Part model, mm, in its own coordinate system. Face numbers are marked on the shaded views. A direction names the side the tool comes from. Round coordinates to 2 decimals unless told otherwise and drop trailing zeros. Loops run counter-clockwise (first coordinate to the right, second up) from the corner with the lowest first, then second, coordinate; pieces in that order, holes last. Notation, with made-up numbers: M 73,73.25 L 100,73.25 A22 cw 100,98.25 Z; hole C 76,-30 d5. An arc over 180 degrees is marked long. Put each result on its own line as item: value. Start each with the question number.
1) Which spindle directions (+Z, -Z, +X, -X, +Y, -Y) get a long thin tool onto all of the face, cutting with end or side? Do the marked faces 5 and 6. Say none if no direction does.
2) Drop flat-ended pins along their axis: pin 1 Ø4 at (x, z) = (42, 7.5) entering from +Y; pin 2 Ø5 at (x, z) = (3, 2) entering from +Y; pin 3 Ø6 at (y, z) = (-1.5, 5.5) entering from +X; pin 4 Ø6.5 at (x, y) = (-64, 10) entering from +Z. Give the stop position or say it passes through.
3) Pull direction Y, two halves, no side cores. Call the marked faces 1, 2, 3 and 4: +Y half, -Y half, draft (parallel to the pull), parting line (faces both ways), or undercut.
4) Slice it at A-A on x = -9.5. Give the cut face in (y, z), then the cut area to 3 significant figures.
5) Probe line 1 along X through (y, z) = (10, 6); line 2 along X through (y, z) = (10, 9.75); line 3 along X through (y, z) = (7.25, 2.25). List the from-to ranges inside material, lowest first.
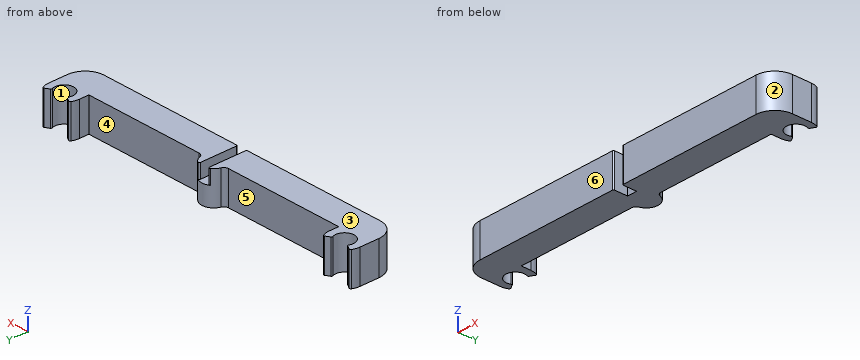
```python
from build123d import *

# Parameters (mm, degrees)
F1_DEPTH = 14
F2_W     = 4.1
F2_H     = 18.371435
F3_DEPTH = 6
F4_R     = 8
F5_R     = 0.5
F6_R     = 2


with BuildPart() as f1:
    # F0 (on Top) → F1 (new body)
    with BuildSketch(Plane.XY):
        with BuildLine():
            Line((-71, -6), (-2.05, -6))
            Line((-2.05, -6), (-2.05, 0))
            Line((-2.05, 0), (-2.05, 6))
            Line((-2.05, 6), (-5, 6))
            Line((-5, 6), (-57, 6))
            Line((-57, 6), (-57, 10))
            ThreePointArc((-57, 10), (-57.238519, 11.811733), (-57.937822, 13.5))
            Line((-57.937822, 13.5), (-60.535898, 12))
            ThreePointArc((-60.535898, 12), (-64, 6), (-67.464102, 12))
            Line((-67.464102, 12), (-70.062178, 13.5))
            ThreePointArc((-70.062178, 13.5), (-70.761481, 11.811733), (-71, 10))
            Line((-71, 10), (-71, 6))
            Line((-71, 6), (-71, -6))
        make_face()
        Polygon((-2.05, 6), (-2.05, 0), (0, 0), (2.05, 0), (2.05, 6), (0, 6), align=None)
        with BuildLine():
            Line((-5, 6), (-2.05, 6))
            Line((-2.05, 6), (0, 6))
            Line((0, 6), (2.05, 6))
            Line((2.05, 6), (5, 6))
            ThreePointArc((5, 6), (0, 11), (-5, 6))
        make_face()
        with BuildLine():
            Line((2.05, 6), (2.05, 0))
            Line((2.05, 0), (2.05, -6))
            Line((2.05, -6), (71, -6))
            Line((71, -6), (71, 6))
            Line((71, 6), (71, 10))
            ThreePointArc((71, 10), (70.761481, 11.811733), (70.062178, 13.5))
            Line((70.062178, 13.5), (67.464102, 12))
            ThreePointArc((67.464102, 12), (64, 6), (60.535898, 12))
            Line((60.535898, 12), (57.937822, 13.5))
            ThreePointArc((57.937822, 13.5), (57.238519, 11.811733), (57, 10))
            Line((57, 10), (57, 6))
            Line((57, 6), (5, 6))
            Line((5, 6), (2.05, 6))
        make_face()
    extrude(amount=F1_DEPTH)

    # F2 (on face) → F3 (cut)
    with BuildSketch(Plane.XY.offset(14)):
        with Locations((0, 9.185717)):
            Rectangle(F2_W, F2_H)
    extrude(amount=-F3_DEPTH, mode=Mode.SUBTRACT)

    # F4
    f4_edges = [f1.edges().sort_by_distance(p)[0] for p in [
        (71, -6, 7),
        (-71, -6, 7),
    ]]
    fillet(f4_edges, radius=F4_R)

    # F5
    f5_edges = [f1.edges().sort_by_distance(p)[0] for p in [
        (2.05, -6, 7),
        (-2.05, -6, 7),
        (-2.05, 10.560428, 11),
        (2.05, 10.560428, 11),
        (-67.464102, 12, 7),
        (-60.535898, 12, 7),
        (60.535898, 12, 7),
        (67.464102, 12, 7),
        (70.062178, 13.5, 7),
        (57.937822, 13.5, 7),
        (-57.937822, 13.5, 7),
        (-70.062178, 13.5, 7),
    ]]
    fillet(f5_edges, radius=F5_R)

    # F6
    f6_edges = [f1.edges().sort_by_distance(p)[0] for p in [
        (-5, 6, 7),
        (5, 6, 7),
    ]]
    fillet(f6_edges, radius=F6_R)


solid = f1.part
```
Recorded:
1. face 5: +Z, -Z, +Y
1. face 6: +Z, -Z, +X, -X, -Y
2. pin 1: stops at y = 6
2. pin 2: stops at y = 10.97
2. pin 3: stops at x = 70.98
2. pin 4: passes through
3. face 1: undercut
3. face 2: -Y half
3. face 3: draft
3. face 4: +Y half
4. outline: M -6,0 L 6,0 L 6,14 L -6,14 Z
4. area: 168 mm2
5. line 1: x = -71 to -68, -60 to -57, -3 to 3, 57 to 60, 68 to 71
5. line 2: x = -71 to -68, -60 to -57, -3 to -2.14, 2.14 to 3, 57 to 60, 68 to 71
5. line 3: x = -71 to -66.9, -61.1 to -57, -4.85 to 4.85, 57 to 61.1, 66.9 to 71
